For this review, take the finished solid that the model builds, in its own axes (mm). A direction names the side the tool comes from. Give positions to 0.01 mm unless a question says otherwise; leave off trailing zeros. Write each loop counter-clockwise with the first axis right and the second up, starting at its lowest first coordinate (ties: lowest second). Pieces come first, ordered by that corner, then holes. Notation, with made-up numbers: (-37, 50.25) -> (11, 50.25) arc R17 ccw to (11, 58.25) -> close; hole circle Ø5 at (-9, -19.75). An arc over 180 degrees is marked (long way). Write item = value, one per line.
```python
from build123d import *

# Parameters (mm, degrees)
SKETCH2_W           = 110
SKETCH2_H           = 75
BASE_DEPTH          = 56
SKETCH3_R           = 5
HV_CONNECTORS_DEPTH = 23
SKETCH4_R           = 10
LV_CONNECTOR_DEPTH  = 51.38
SKETCH5_W           = 10
SKETCH5_H           = 10
HV_CONNECTOR_DEPTH  = 10


with BuildPart() as part:
    # Sketch2 → Base (new body)
    with BuildSketch(Plane(origin=(0, 0, 0), x_dir=(1, 0, 0), z_dir=(0, 1, 0))):
        Rectangle(SKETCH2_W, SKETCH2_H)
    extrude(amount=BASE_DEPTH)

    # Sketch3 → HV- Connectors (add)
    with BuildSketch(Plane(origin=(0, 56, 0), x_dir=(1, 0, 0), z_dir=(0, 1, 0))):
        with Locations((30, 0)):
            Circle(SKETCH3_R)
        with Locations((-30, 0)):
            Circle(SKETCH3_R)
    extrude(amount=HV_CONNECTORS_DEPTH)

    # Sketch4 → LV Connector (add)
    with BuildSketch(Plane.ZY.offset(55)):
        with Locations((0, 25)):
            Circle(SKETCH4_R)
    extrude(amount=LV_CONNECTOR_DEPTH)

    # Sketch5 → HV+ Connector (add)
    with BuildSketch(Plane(origin=(0, 56, 0), x_dir=(1, 0, 0), z_dir=(0, 1, 0))):
        with Locations((-30, -22.5)):
            Rectangle(SKETCH5_W, SKETCH5_H)
    extrude(amount=HV_CONNECTOR_DEPTH)


solid = part.part
```
(1) To check wall thickness, follow probe 1 along Y at (x, z) = (9, -9); probe 2 along Y at (x, z) = (-31, 23.5); probe 3 along X at (y, z) = (55, 3.5). State the ranges of each line that lie inside material, in increasing order.
Answers below:
probe_1 = 0 to 56
probe_2 = 0 to 66
probe_3 = -55 to 55
(2) Take a section at D-D (x = -30). Write out the cut boundary in (y, z).
Answers below:
outline = (0, -37.5) -> (56, -37.5) -> (56, -5) -> (79, -5) -> (79, 5) -> (56, 5) -> (56, 17.5) -> (66, 17.5) -> (66, 27.5) -> (56, 27.5) -> (56, 37.5) -> (0, 37.5) -> close
(3) The part is to be moulded in two halves that separate along Z. For faces 1 (the face through (-30, 61, 17.5)), 2 (the face through (25, 67, 0)), 3 (the face through (-1, 28, -37.5)), 4 (the face through (-1, 28, 37.5)), say which applies: released by +Z, released by -Z, zero draft, split by the parting line, or undercut.
Answers below:
face_1 = undercut
face_2 = split by the parting line
face_3 = released by -Z
face_4 = released by +Z
(4) Tool access review of faces 5 (the face through (-30, 66, 22)), 6 (the face through (-35, 67, 0)), 7 (the face through (-25, 61, 23)), 8 (the face through (-35, 61, 23)): name each direction out of +Z, -Z, +X, -X, +Y, -Y from which nothing blocks a thin tool from reaching the whole face with its end or side.
Answers below:
face_5 = +Z, +X, -X, +Y
face_6 = +Y
face_7 = +Z, -Z, +X, +Y
face_8 = +Z, -Z, -X, +Y
(5) Take a section at B-B (y = 25). Write out the cut boundary in (x, z).
Answers below:
outline = (-106.38, -10) -> (-55, -10) -> (-55, -37.5) -> (55, -37.5) -> (55, 37.5) -> (-55, 37.5) -> (-55, 10) -> (-106.38, 10) -> close
(6) Take a section at A-A (z = 0). Write out the cut boundary in (x, y), plus the area to 3 significant figures.
Answers below:
outline = (-106.38, 15) -> (-55, 15) -> (-55, 0) -> (55, 0) -> (55, 56) -> (35, 56) -> (35, 79) -> (25, 79) -> (25, 56) -> (-25, 56) -> (-25, 79) -> (-35, 79) -> (-35, 56) -> (-55, 56) -> (-55, 35) -> (-106.38, 35) -> close
area = 7,650 mm^2
(7) For pin 1 (8 mm diameter, centred on x = -30, y = 61, fed in from -Z); pin 2 (10 mm diameter, centred on x = -84.5, y = 26.5, fed in from -Z); pin 3 (5 mm diameter, centred on x = -90, z = 4.5, fed in from +Y); pin 4 (11 mm diameter, centred on y = 61, z = 24, fed in from +X), all flat-tipped, find the tip position at first contact; note any pin that passes through.
Answers below:
pin_1 = -5
pin_2 = -10
pin_3 = 34.8
pin_4 = 55
(8) Take a section at C-C (x = 30). Write out the cut boundary in (y, z).
Answers below:
outline = (0, -37.5) -> (56, -37.5) -> (56, -5) -> (79, -5) -> (79, 5) -> (56, 5) -> (56, 37.5) -> (0, 37.5) -> close
